```python
from build123d import *

# Parameters (mm, degrees)
SKETCH2_R               = 3
CUT_EXTRUDE1_DEPTH      = 10
CUT_EXTRUDE1_DEPTH_BACK = 10
FILLET1_R               = 1
FILLET2_R               = 2
SKETCH3_R               = 1.5
CUT_EXTRUDE2_DEPTH      = 6


with BuildPart() as part:
    # Sketch1 → Revolve1 (revolve)
    with BuildSketch(Plane.XY):
        Polygon((0, 0), (0, 6.325), (15, 6.325), (20.6, 3.165), (86.95, 3.165), (88.3, 1.875), (104, 1.875), (106.6, 0), align=None)
    revolve(axis=Axis((106.6, 0, 0), (-1, 0, 0)))

    # Sketch2 → Cut-Extrude1 (cut, two sides)
    with BuildSketch(Plane(origin=(0, 0, 0), x_dir=(1, 0, 0), z_dir=(0, 1, 0))) as cut_extrude1_sk:
        with Locations((5, 0)):
            Circle(SKETCH2_R)
    extrude(amount=CUT_EXTRUDE1_DEPTH, mode=Mode.SUBTRACT)
    extrude(cut_extrude1_sk.sketch, amount=-CUT_EXTRUDE1_DEPTH_BACK, mode=Mode.SUBTRACT)

    # Fillet1
    fillet1_edges = [part.edges().sort_by_distance(p)[0] for p in [
        (0, -6.325, 0),
    ]]
    fillet(fillet1_edges, radius=FILLET1_R)

    # Fillet2
    fillet2_edges = [part.edges().sort_by_distance(p)[0] for p in [
        (15, -6.325, 0),
        (20.6, -3.165, 0),
    ]]
    fillet(fillet2_edges, radius=FILLET2_R)

    # Sketch3 → Cut-Extrude2 (cut)
    with BuildSketch(Plane.ZY):
        Circle(SKETCH3_R)
    extrude(amount=-CUT_EXTRUDE2_DEPTH, mode=Mode.SUBTRACT)


solid = part.part
```
Model file for the job. Use its own axes, mm. A direction names the side the tool comes from. Coordinates: 2 decimals unless noted, no trailing zeros. Order: outer loops, then holes, each group sorted by start corner. A loop starts at its lowest first (then second) coordinate and runs counter-clockwise, first axis right, second up. Notation, with made-up numbers: (49.25, 10) -> (73.25, 10) arc R16 ccw to (73.25, 22) -> close; hole circle Ø9 at (26.25, 50). An arc over 180 degrees is marked (long way). Answer as a JSON object with one key per item and string values. Group by question number.
1) Which spindle directions (+Z, -Z, +X, -X, +Y, -Y) get a long thin tool onto all of the face, cutting with end or side? Do faces 1 (the face through (7.832, -4.662, -4.275)), 2 (the face through (54.5, 3.02, -0.95)). Say none if no direction does.
2) Flat gauge pins, fed straight in: pin 1 (2 mm diameter, centred on x = 60.5, z = -3, fed in from -Y); pin 2 (2 mm diameter, centred on x = 19.5, y = 2.5, fed in from -Z); pin 3 (4 mm diameter, centred on y = -3, z = 2, fed in from +X); pin 4 (5.5 mm diameter, centred on x = 5, z = 0, fed in from -Y). Where does each tip first touch, or does it go through?
3) Pull direction Y, two halves, no side cores. Call faces 3 (the face through (96.26, -1.873, -0.082)), 4 (the face through (1.184, -0.575, 1.386)), 5 (the face through (0, 1.3, 1.1)): +Y half, -Y half, draft (parallel to the pull), parting line (faces both ways), or undercut.
4) Drill centre lines: L1, parallel to Z at x = 0.85, y = 0; L2, parallel to Y at x = 42, z = -1; L3, parallel to X at y = 3.5, z = 0. Where is each one in solid material? Low to high.
5) Cut at B-B, the plane x = 99.5. Write the cut outline in (y, z) (3 decimals), then the cut area to 3 significant figures.
6) Cut at A-A, the plane x = 5. Write the cut outline in (y, z) (3 decimals).
7) Cut at C-C, the plane x = 47.5. Write the cut outline in (y, z) (3 decimals), then the cut area to 3 significant figures.
Check values:
{
 "1": {"face 1": "+X, -X", "face 2": "+X"},
 "2": {"pin 1": "stops at y = -2.45", "pin 2": "stops at z = -3.79", "pin 3": "stops at x = 104.37", "pin 4": "passes through"},
 "3": {"face 3": "parting line", "face 4": "undercut", "face 5": "draft"},
 "4": {"L1": "z = -6.31 to -1.5, 1.5 to 6.31", "L2": "y = -3 to 3", "L3": "x = 0 to 2, 8 to 20.01"},
 "5": {"outline": "circle Ø3.75 at (0, 0)", "area": "11.0 mm²"},
 "6": {"outline": "(-5.568, -3) arc R6.325 ccw to (5.568, -3) -> close; (-5.568, 3) -> (5.568, 3) arc R6.325 ccw to start"},
 "7": {"outline": "circle Ø6.33 at (0, 0)", "area": "31.5 mm²"}
}
